Work out the finished part from the listing and answer in its coordinate system (mm). Face numbers are marked on the shaded views. A direction names the side the tool comes from. Coordinates: 2 decimals unless noted, no trailing zeros. Write each loop counter-clockwise with the first axis right and the second up, starting at its lowest first coordinate (ties: lowest second). Pieces come first, ordered by that corner, then holes. Notation, with made-up numbers: (-0.5, 12) - (26.5, 12) arc R22 cw to (26.5, 21) - close; hole circle Ø2 at (66, 53.5). An arc over 180 degrees is marked (long way). Use one line per item in the form item = value. Start each with the question number.
Item 1: Determine the mould class of the marked faces 6, 7 and 8 for opening direction X: released by +X, released by -X, zero draft, split by the parting line, or undercut.
Item 2: A cutting plane is placed at C-C (z = 11.75). Write down the section's boundary in (x, y).
Item 3: Given pin 1 (4.5 mm diameter, centred on y = 24.5, z = 12.5, fed in from -X); pin 2 (3.5 mm diameter, centred on y = 33, z = 14, fed in from +X); pin 3 (1 mm diameter, centred on x = 69, z = 14, fed in from +Y), each flat-ended and moving along its own axis, determine where each tip first touches the part or whether it passes through.
Item 4: A cutting plane is placed at D-D (y = 40). Write down the section's boundary in (x, z).
Item 5: A cutting plane is placed at A-A (y = 16). Write down the section's boundary in (x, z), then the cut area to 3 significant figures.
Item 6: Consider probe 1 along X at (y, z) = (24, 10.25); probe 2 along Z at (x, y) = (73, 17.5); probe 3 along Y at (x, z) = (49, 10.25). Determine where each line is inside the solid, lowest interval first.
Item 7: A cutting plane is placed at B-B (x = 32). Write down the section's boundary in (y, z), then the cut area to 3 significant figures.
Item 8: For the marked faces 1, 2, 3, 4 and 5, determine the directions among +Z, -Z, +X, -X, +Y, -Y from which every point of the face is accessible in a straight line to the end or side of a thin tool.
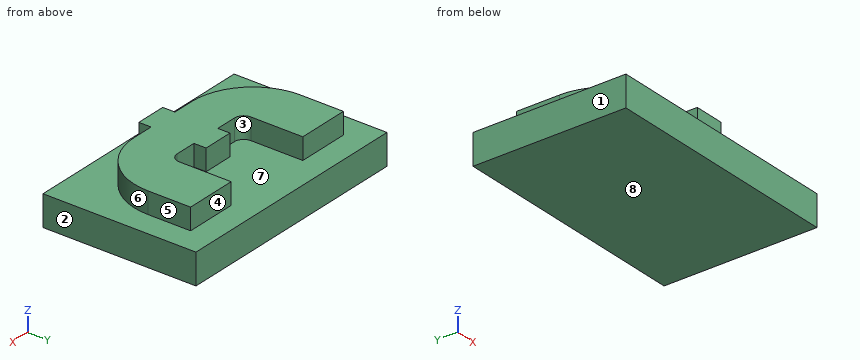
from build123d import *

# Parameters (mm, degrees)
SKETCH1_W           = 80
SKETCH1_H           = 50
BOSS_EXTRUDE1_DEPTH = 10
SKETCH2_W           = 64
SKETCH2_H           = 34
BOSS_EXTRUDE2_DEPTH = 7
FILLET1_R           = 20
SKETCH3_W           = 10
SKETCH3_H           = 7
BOSS_EXTRUDE3_DEPTH = 4
SKETCH4_W           = 30
SKETCH4_H           = 20
CUT_EXTRUDE1_DEPTH  = 7
FILLET2_R           = 3
SKETCH5_W           = 10
SKETCH5_H           = 7
BOSS_EXTRUDE4_DEPTH = 4


with BuildPart() as part:
    # Sketch1 → Boss-Extrude1 (new body)
    with BuildSketch(Plane.XY):
        with Locations((40, 25)):
            Rectangle(SKETCH1_W, SKETCH1_H)
    extrude(amount=BOSS_EXTRUDE1_DEPTH)

    # Sketch2 → Boss-Extrude2 (add)
    with BuildSketch(Plane.XY.offset(10)):
        with Locations((40, 25)):
            Rectangle(SKETCH2_W, SKETCH2_H)
    extrude(amount=BOSS_EXTRUDE2_DEPTH)

    # Fillet1
    fillet1_edges = [part.edges().sort_by_distance(p)[0] for p in [
        (8, 8, 13.5),
        (72, 8, 13.5),
    ]]
    fillet(fillet1_edges, radius=FILLET1_R)

    # Sketch3 → Boss-Extrude3 (add)
    with BuildSketch(Plane(origin=(0, 8, 0), x_dir=(-1, 0, 0), z_dir=(0, -1, 0))):
        with Locations((-40, -13.5)):
            Rectangle(SKETCH3_W, SKETCH3_H)
    extrude(amount=BOSS_EXTRUDE3_DEPTH)

    # Sketch4 → Cut-Extrude1 (cut)
    with BuildSketch(Plane.XY.offset(17)):
        with Locations((40, 32)):
            Rectangle(SKETCH4_W, SKETCH4_H)
    extrude(amount=-CUT_EXTRUDE1_DEPTH, mode=Mode.SUBTRACT)

    # Fillet2
    fillet2_edges = [part.edges().sort_by_distance(p)[0] for p in [
        (55, 22, 13.5),
        (25, 22, 13.5),
    ]]
    fillet(fillet2_edges, radius=FILLET2_R)

    # Sketch5 → Boss-Extrude4 (add)
    with BuildSketch(Plane(origin=(0, 22, 0), x_dir=(1, 0, 0), z_dir=(0, 1, 0))):
        with Locations((40, -13.5)):
            Rectangle(SKETCH5_W, SKETCH5_H)
    extrude(amount=BOSS_EXTRUDE4_DEPTH)


solid = part.part
Answer:
q1.face_6 = released by +X
q1.face_7 = undercut
q1.face_8 = zero draft
q2.outline = (8, 28) arc R20 ccw to (28, 8) - (35, 8) - (35, 4) - (45, 4) - (45, 8) - (52, 8) arc R20 ccw to (72, 28) - (72, 42) - (55, 42) - (55, 25) arc R3 cw to (52, 22) - (45, 22) - (45, 26) - (35, 26) - (35, 22) - (28, 22) arc R3 cw to (25, 25) - (25, 42) - (8, 42) - close
q3.pin_1 = 8.04
q3.pin_2 = 72
q3.pin_3 = 42
q4.outline = (0, 0) - (80, 0) - (80, 10) - (72, 10) - (72, 17) - (55, 17) - (55, 10) - (25, 10) - (25, 17) - (8, 17) - (8, 10) - (0, 10) - close
q5.outline = (0, 0) - (80, 0) - (80, 10) - (68, 10) - (68, 17) - (12, 17) - (12, 10) - (0, 10) - close
q5.area = 1,190 mm²
q6.probe_1 = 8.4 to 25.17, 35 to 45, 54.83 to 71.6
q6.probe_2 = 0 to 10
q6.probe_3 = 8 to 22
q7.outline = (0, 0) - (50, 0) - (50, 10) - (22, 10) - (22, 17) - (8, 17) - (8, 10) - (0, 10) - close
q7.area = 598 mm²
q8.face_1 = +Z, -Z, -X, +Y, -Y
q8.face_2 = +Z, -Z, +X, +Y, -Y
q8.face_3 = +Z, +Y
q8.face_4 = +Z, +X, -X, +Y
q8.face_5 = +Z, +X, +Y, -Y
